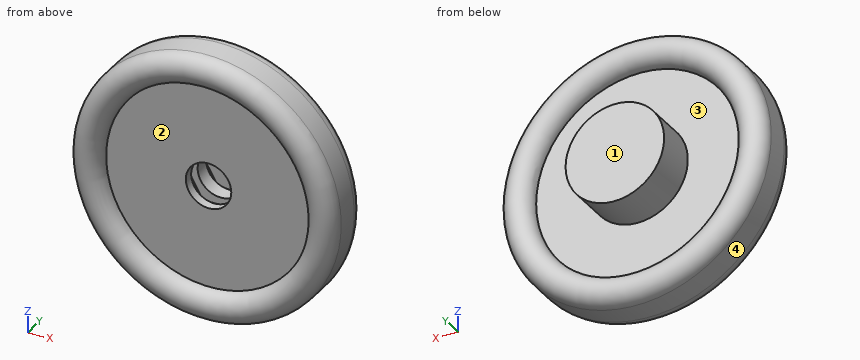
```python
from build123d import *

# Parameters (mm, degrees)
SKETCH_1_W          = 13.5
SKETCH_1_H          = 3
SKETCH_4_R          = 6.5
EXTRUDE_1_DEPTH     = 7
CUT_EXTRUDE_1_DEPTH = 1.5
CUT_EXTRUDE_START   = 3.5
CUT_EXTRUDE_2_DEPTH = 1.5
SKETCH_6_R          = 3
CUT_EXTRUDE_3_DEPTH = 6.25


with BuildPart() as part:
    # Эскиз1 → Повернуть1 (revolve)
    with BuildSketch(Plane.XY):
        with BuildLine():
            Line((17.5, -1.5), (17.5, 1.5))
            ThreePointArc((17.5, 1.5), (15.5, 3.5), (13.5, 1.5))
            Line((13.5, 1.5), (13.5, -1.5))
            ThreePointArc((13.5, -1.5), (15.5, -3.5), (17.5, -1.5))
        make_face()
        with Locations((6.75, 0)):
            Rectangle(SKETCH_1_W, SKETCH_1_H)
    revolve(axis=Axis((0, 0, 0), (0, -1, 0)))

    # Эскиз4 → Бобышка-Вытянуть1 (add)
    with BuildSketch(Plane(origin=(0, 0, 0), x_dir=(1, 0, 0), z_dir=(0, 1, 0))):
        Circle(SKETCH_4_R)
    extrude(amount=EXTRUDE_1_DEPTH)

    # Эскиз5 → Вырез-Вытянуть1 (cut)
    with BuildSketch(Plane(origin=(0, 4.75, 0), x_dir=(-1, 0, 0), z_dir=(0, -1, 0))):
        Polygon((2.309401077, 4), (-2.309401077, 4), (-4.618802154, 0), (-2.309401077, -4), (2.309401077, -4), (4.618802154, 0), align=None)
    extrude(amount=CUT_EXTRUDE_1_DEPTH, mode=Mode.SUBTRACT)

    # Эскиз5<2> → Вырез-Вытянуть2 (cut)
    with BuildSketch(Plane(origin=(0, 4.75, 0), x_dir=(-1, 0, 0), z_dir=(0, -1, 0)).offset(CUT_EXTRUDE_START)):
        Polygon((2.309401077, 4), (-2.309401077, 4), (-4.618802154, 0), (-2.309401077, -4), (2.309401077, -4), (4.618802154, 0), align=None)
    extrude(amount=CUT_EXTRUDE_2_DEPTH, mode=Mode.SUBTRACT)

    # Эскиз6 → Вырез-Вытянуть3 (cut)
    with BuildSketch(Plane.XZ.offset(1.5)):
        Circle(SKETCH_6_R)
    extrude(amount=-CUT_EXTRUDE_3_DEPTH, mode=Mode.SUBTRACT)


solid = part.part
```
The listing builds one solid part. Answer for the finished solid, in the listing's coordinates (mm). Face numbers are marked on the shaded views. Round coordinates to 2 decimals unless told otherwise and drop trailing zeros. Loops run counter-clockwise (first coordinate to the right, second up) from the corner with the lowest first, then second, coordinate; pieces in that order, holes last. Notation, with made-up numbers: (22, 73.5) - (69, 73.5) arc R26 cw to (69, 98.5) - close; hole circle Ø3 at (66.25, -26.75). An arc over 180 degrees is marked (long way). Use one line per item in the form item = value. Start each with the question number.
1. The part is cut by section A-A on x = 0. Determine the outline of the cut face in (y, z), then the cut area to 3 significant figures.
2. Given pin 1 Ø4 at (x, z) = (-11, 6.5) entering from -Y; pin 2 Ø2 at (x, y) = (-2.5, 3.5) entering from +Z; pin 3 Ø6 at (y, z) = (-2.5, -6) entering from -X, each flat-ended and moving along its own axis, determine where each tip first touches the part or whether it passes through.
3. The part is cut by section C-C on z = 3.5. Give the number of separate pieces and of enclosed holes in the cut face, then the cut area to 3 significant figures.
4. The part is cut by section B-B on y = -1. Determine the outline of the cut face in (x, z), then the cut area to 3 significant figures.
5. Consider line 1 (Z direction, x = 0, y = -0.95); line 2 (Z direction, x = 0, y = 2.7); line 3 (Z direction, x = 0, y = 1.95). Determine where each line is inside the solid, lowest interval first. Write a range as [from, to].
6. For a pull along X with two mould halves and no side action, classify the marked faces 1, 2, 3 and 4 as pulls with the +X half, pulls with the -X half, needs draft (parallel to the pull), parting line crosses it, or undercut.
Geometry check:
q1.outline = (-1.5, -17.5) - (1.5, -17.5) arc R2 ccw to (1.5, -13.5) - (1.5, -6.5) - (7, -6.5) - (7, 6.5) - (1.5, 6.5) - (1.5, 13.5) arc R2 ccw to (1.5, 17.5) - (-1.5, 17.5) arc R2 ccw to (-1.5, 13.5) - (-1.5, 3) - (-0.25, 3) - (-0.25, 4) - (1.25, 4) - (1.25, 3) - (3.25, 3) - (3.25, 4) - (4.75, 4) - (4.75, -4) - (3.25, -4) - (3.25, -3) - (1.25, -3) - (1.25, -4) - (-0.25, -4) - (-0.25, -3) - (-1.5, -3) - (-1.5, -13.5) arc R2 ccw to start
q1.area = 158 mm^2
q2.pin_1 = -3.36
q2.pin_2 = 17.07
q2.pin_3 = -17.21
q3.separate_pieces = 1
q3.enclosed_holes = 2
q3.area = 173 mm^2
q4.outline = circle Ø35 at (0, 0); hole circle Ø6 at (0, 0)
q4.area = 934 mm^2
q5.line_1 = [-17.5, -3], [3, 17.5]
q5.line_2 = [-17.1, -13.9], [-6.5, -3], [3, 6.5], [13.9, 17.1]
q5.line_3 = [-17.45, -13.55], [-6.5, -3], [3, 6.5], [13.55, 17.45]
q6.face_1 = needs draft
q6.face_2 = undercut
q6.face_3 = undercut
q6.face_4 = parting line crosses it
